Autodesk Inventor part; units mm, degrees
ref_plane "YZ Plane" through (0, 0, 0) normal (1, 0, 0) x (0, 1, 0)
ref_plane "XZ Plane" through (0, 0, 0) normal (0, 1, 0) x (-1, 0, 0)
ref_plane "XY Plane" through (0, 0, 0) normal (0, 0, 1) x (1, 0, 0)
sketch "Sketch1" plane through (0, 0, 0) normal (0, 0, 1) x (1, 0, 0)
  point P0 (0, 0)
sketch "Sketch2" plane through (0, 0, 0) normal (0, 0, 1) x (1, 0, 0)
  line L0 (-69, 0) -> (-69, 4)
  line L1 (-69, 4) -> (-54, 4)
  line L2 (-54, 4) -> (-54, 36)
  line L3 (-54, 36) -> (0, 36)
  line L4 (0, 36) -> (0, 34)
  line L5 (0, 34) -> (-51.5, 34)
  line L6 (-51.5, 34) -> (-51.5, 0)
  line L7 (-51.5, 0) -> (-69, 0)
  point P0 (0, 0)
  point P1 (-25.75, 34)
  point P2 (0, 35)
  dimension "d0" = 2
  dimension "d1" = 2.5
  dimension "d2" = 4
  dimension "d3" = 4
  dimension "d4" = 15
  dimension "d6" = 0
  dimension "d8" = 51.5
  dimension "d11" = 34
extrude "Extrusion1" add sketch "Sketch2" along normal mid plane 10
mirror "Mirror1" about plane through (0, 34, 0) normal (1, 0, 0) of "Extrusion1"
sketch "Sketch3" plane through (0, 0, 5) normal (0, 0, 1) x (1, 0, 0)
  line L0 (-54, 36) -> (-54, 4)
  line L1 (-54, 36) -> (-54, 4)
  line L2 (-54, 4) -> (-69, 4)
  line L3 (-54, 4) -> (-69, 4)
  line L4 (-69, 4) -> (-54, 36)
  point P0 (0, 0)
extrude "Extrusion2" add sketch "Sketch3" against normal blind 1
mirror "Mirror2" about plane through (0, 0, 0) normal (1, 0, 0) of "Extrusion2"
sketch "Sketch4" plane through (54, 4, -5) normal (0, 1, 0) x (1, 0, 0)
  circle A0 centre (7.5, -4.5) radius 1.9938
  line L0 (0, 0) -> (0, -9)
  line L1 (15, 0) -> (0, 0)
  point P0 (-54, -5)
  point P1 (0, -4.5)
  dimension "d14" = 7.5
  dimension "d15" = 4.5
extrude "Extrusion3" cut sketch "Sketch4" against normal blind 20
mirror "Mirror3" about plane through (0, 0, 0) normal (1, 0, 0) of "Extrusion3"
equation "\"d3\" = d2"
properties part number "KVMMount"
Build history of the part. All positions in model axes, mm. A direction names the side the tool comes from. Give positions to 0.01 mm unless a question says otherwise; leave off trailing zeros. Order: outer loops, then holes, each group sorted by start corner. A loop starts at its lowest first (then second) coordinate and runs counter-clockwise, first axis right, second up. Notation, with made-up numbers: M 86,46 L 129,46 A13 ccw 129,65 Z; hole C 29.25,9 d7. An arc over 180 degrees is marked long. Use one line per item in the form item = value.
Q1. Pull direction X, two halves, no side cores. Call faces 1 (the flat face through (-51.5, 17, 0)), 2 (the flat face through (58, 13, 4)), 3 (the flat face through (-69, 2, 0)), 4 (the flat face through (54, 20, -1)): released by +X, released by -X, zero draft, split by the parting line, or undercut.
Conclusion:
face_1 = undercut
face_2 = zero draft
face_3 = released by -X
face_4 = released by +X
Q2. Slice it at A-A, the plane x = 61.5. Write the cut outline in (y, z).
Conclusion:
outline = M 0,-5 L 4,-5 L 4,-2.49 L 0,-2.49 Z; M 0,1.49 L 4,1.49 L 4,4 L 20,4 L 20,5 L 0,5 Z
Q3. Slice it at C-C, the plane y = 19. Write the cut outline in (x, z).
Conclusion:
outline = M -61.97,4 L -54,4 L -54,-5 L -51.5,-5 L -51.5,5 L -61.97,5 Z; M 51.5,-5 L 54,-5 L 54,4 L 61.97,4 L 61.97,5 L 51.5,5 Z
Q4. Slice it at B-B, the plane z = -0.5. Write the cut outline in (x, y), and give its area (3 significant figures).
Conclusion:
outline = M -69,0 L -63.49,0 L -63.49,4 L -69,4 Z; M -59.51,0 L -51.5,0 L -51.5,34 L 51.5,34 L 51.5,0 L 59.51,0 L 59.51,4 L 54,4 L 54,36 L -54,36 L -54,4 L -59.51,4 Z; M 63.49,0 L 69,0 L 69,4 L 63.49,4 Z
area = 474 mm2
Q5. Slice it at D-D, the plane x = -0.5. Write the cut outline in (y, z), and give its area (3 significant figures).
Conclusion:
outline = M 34,-5 L 36,-5 L 36,5 L 34,5 Z
area = 20.0 mm2
Q6. Wall check: probe 1 along X at (y, z) = (2.8, -0.5); probe 2 along X at (y, z) = (17, 2); probe 3 along Y at (x, z) = (44, -2.75). Give the ranges that are in metal, low to high.
Conclusion:
probe_1 = -69 to -63.49, -59.51 to -51.5, 51.5 to 59.51, 63.49 to 69
probe_2 = -54 to -51.5, 51.5 to 54
probe_3 = 34 to 36
Q7. Pin check, flat tips, straight feed: P1, Ø2.5, axis at x = -60, z = 1, coming from the +Y side; P2, Ø6, axis at x = 28.5, z = -2, coming from the -Y side; P3, Ø4.5, axis at x = 59, y = 28, coming from the -Z side; P4, Ø3, axis at x = 61.5, z = -0.5, coming from the -Y side. Stop position of each tip, or through.
Conclusion:
P1 = 4
P2 = 34
P3 = 4
P4 = through
Q8. Which spindle directions (+Z, -Z, +X, -X, +Y, -Y) get a long thin tool onto all of the face, cutting with end or side? Do faces 5 (the flat face through (1, 34, 0)), 6 (the flat face through (-54, 20, -1)), 7 (the flat face through (61.395, 20.224, 4.507)), 8 (the flat face through (61, 4, -3)), 9 (the flat face through (69, 2, 0)). Say none if no direction does.
Conclusion:
face_5 = +Z, -Z, -Y
face_6 = -Z, -X, +Y
face_7 = +Z, -Z, +X, +Y
face_8 = -Z, +X, +Y
face_9 = +Z, -Z, +X, +Y, -Y
